```python
from build123d import *

# Parameters (mm, degrees)
EXTRUDE_1_DEPTH      = 3
EXTRUDE_1_DEPTH_BACK = 3
SKETCH_1_W           = 34
SKETCH_1_H           = 70
SKETCH_3_W           = 34
SKETCH_3_H           = 230
EXTRUDE_2_DEPTH      = 5
SKETCH_4_W           = 34
SKETCH_4_H           = 5
EXTRUDE_3_DEPTH      = 30
EXTRUDE_START        = -5
EXTRUDE_4_OUTLINE_W  = 34
EXTRUDE_4_OUTLINE_H  = 25
EXTRUDE_4_DEPTH      = 5
SKETCH_7_R           = 2.2
CUT_EXTRUDE_1_DEPTH  = 139.343774706
SKETCH_9_R           = 3.25
CUT_EXTRUDE_3_DEPTH  = 126.749751491
EXTRUDE_5_DEPTH      = 34
SKETCH_12_W          = 37
SKETCH_12_H          = 52.36766615
CUT_EXTRUDE_5_DEPTH  = 139.343774706
EXTRUDE_START_2      = 3.5
SKETCH_13_W          = 12
SKETCH_13_H          = 10
SKETCH_13_W_2        = 10
SKETCH_13_H_2        = 9
SKETCH_13_R          = 2.2
EXTRUDE_6_DEPTH      = 3.5
EXTRUDE_START_3      = 1.5
SKETCH_14_W          = 10
SKETCH_14_H          = 9
SKETCH_14_R          = 2.2
EXTRUDE_7_DEPTH      = 1.5
SKETCH_15_W          = 7
SKETCH_15_H          = 10
SKETCH_15_R          = 1.9
EXTRUDE_8_DEPTH      = 5
FILLET_2_R           = 15
FILLET_3_R           = 4
FILLET_4_R           = 3
FILLET_5_R           = 6
FILLET_6_R           = 1


# Read off the part's stored shape, not the designer's step: 凸台-拉伸4
with BuildPart() as part:
    # 草图1 → 凸台-拉伸1 (new, two sides: drawn at the far end of the back side and taken through both)
    with BuildSketch(Plane(origin=(0, 0, 0), x_dir=(1, 0, 0), z_dir=(0, 1, 0)).offset(-EXTRUDE_1_DEPTH_BACK)):
        Rectangle(SKETCH_1_W, SKETCH_1_H)
    extrude(amount=EXTRUDE_1_DEPTH + EXTRUDE_1_DEPTH_BACK)

    # 草图3 → 凸台-拉伸2 (add)
    with BuildSketch(Plane.XY.offset(35)):
        Rectangle(SKETCH_3_W, SKETCH_3_H)
    extrude(amount=EXTRUDE_2_DEPTH)

    # 草图4 → 凸台-拉伸3 (add)
    with BuildSketch(Plane.XZ.offset(3)):
        with Locations((0, 7.5)):
            Rectangle(SKETCH_4_W, SKETCH_4_H)
    extrude(amount=EXTRUDE_3_DEPTH)

    # 凸台-拉伸4 outline → 凸台-拉伸4 (add)
    with BuildSketch(Plane.XZ.offset(33).offset(EXTRUDE_START)):
        with Locations((0, 22.5)):
            Rectangle(EXTRUDE_4_OUTLINE_W, EXTRUDE_4_OUTLINE_H)
    extrude(amount=EXTRUDE_4_DEPTH)

    # 草图7 → 切除-拉伸1 (cut, through all)
    with BuildSketch(Plane.XY.offset(40)):
        with Locations((0, -105)):
            Circle(SKETCH_7_R)
        with Locations((0, 105)):
            Circle(SKETCH_7_R)
    extrude(amount=-CUT_EXTRUDE_1_DEPTH, mode=Mode.SUBTRACT)

    # 草图9 → 切除-拉伸3 (cut, through all)
    with BuildSketch(Plane.XZ.offset(3)):
        with Locations(Location((10, -15, 0), (0, 0, 270))):
            Circle(SKETCH_9_R)
        with Locations(Location((-10, -15, 0), (0, 0, 270))):
            Circle(SKETCH_9_R)
    extrude(amount=-CUT_EXTRUDE_3_DEPTH, mode=Mode.SUBTRACT)

    # 草图10 → 凸台-拉伸5 (add)
    with BuildSketch(Plane(origin=(17, 0, 0), x_dir=(0, 0, -1), z_dir=(1, 0, 0))):
        Polygon((-35, 51.819660113), (-35, 63), (-5, 3), (-10.590169944, 3), align=None)
    extrude(amount=-EXTRUDE_5_DEPTH)

    # 草图12 → 切除-拉伸5 (cut, through all)
    with BuildSketch(Plane.XY.offset(40)):
        with Locations((-1.5, -96.183833075)):
            Rectangle(SKETCH_12_W, SKETCH_12_H)
    extrude(amount=-CUT_EXTRUDE_5_DEPTH, mode=Mode.SUBTRACT)

    # 草图13 → 凸台-拉伸6 (add)
    # profile 1 of 3: a face of its own
    with BuildSketch(Plane.XY.offset(40).offset(EXTRUDE_START_2)):
        with Locations((0, -65)):
            Rectangle(SKETCH_13_W, SKETCH_13_H)
    # profile 2 of 3: a face of its own
    with BuildSketch(Plane.XY.offset(40).offset(EXTRUDE_START_2)):
        with Locations((0, 22)):
            Rectangle(SKETCH_13_W, SKETCH_13_H)
    # profile 3 of 3: a face of its own
    with BuildSketch(Plane.XY.offset(40).offset(EXTRUDE_START_2)):
        with Locations((0, 105)):
            Rectangle(SKETCH_13_W_2, SKETCH_13_H_2)
        with Locations((0, 105)):
            Circle(SKETCH_13_R, mode=Mode.SUBTRACT)
    extrude(amount=-EXTRUDE_6_DEPTH)

    # 草图14 → 凸台-拉伸7 (add)
    with BuildSketch(Plane.XY.offset(43.5).offset(EXTRUDE_START_3)):
        with Locations((0, 105)):
            Rectangle(SKETCH_14_W, SKETCH_14_H)
        with Locations((0, 105)):
            Circle(SKETCH_14_R, mode=Mode.SUBTRACT)
    extrude(amount=-EXTRUDE_7_DEPTH)

    # 草图15 → 凸台-拉伸8 (add)
    # profile 1 of 4: a face of its own
    with BuildSketch(Plane.XY.offset(40)):
        with Locations((-9.5, 22)):
            Rectangle(SKETCH_15_W, SKETCH_15_H)
        with Locations((-9.5, 22)):
            Circle(SKETCH_15_R, mode=Mode.SUBTRACT)
    # profile 2 of 4: a face of its own
    with BuildSketch(Plane.XY.offset(40)):
        with Locations((-9.5, -65)):
            Rectangle(SKETCH_15_W, SKETCH_15_H)
        with Locations((-9.5, -65)):
            Circle(SKETCH_15_R, mode=Mode.SUBTRACT)
    # profile 3 of 4: a face of its own
    with BuildSketch(Plane.XY.offset(40)):
        with Locations((9.5, 22)):
            Rectangle(SKETCH_15_W, SKETCH_15_H)
        with Locations(Location((9.5, 22, 0), (0, 0, 180))):
            Circle(SKETCH_15_R, mode=Mode.SUBTRACT)
    # profile 4 of 4: a face of its own
    with BuildSketch(Plane.XY.offset(40)):
        with Locations((9.5, -65)):
            Rectangle(SKETCH_15_W, SKETCH_15_H)
        with Locations(Location((9.5, -65, 0), (0, 0, 180))):
            Circle(SKETCH_15_R, mode=Mode.SUBTRACT)
    extrude(amount=EXTRUDE_8_DEPTH)

    # 圆角2
    fillet_2_edges = [part.edges().sort_by_distance(p)[0] for p in [
        (17, 115, 37.5),
        (-17, 115, 37.5),
        (-17, 0, -35),
        (17, 0, -35),
    ]]
    fillet(fillet_2_edges, radius=FILLET_2_R)

    # 圆角3
    fillet_3_edges = [part.edges().sort_by_distance(p)[0] for p in [
        (-17, -70, 37.5),
        (17, -70, 37.5),
    ]]
    fillet(fillet_3_edges, radius=FILLET_3_R)

    # 圆角4
    fillet_4_edges = [part.edges().sort_by_distance(p)[0] for p in [
        (0, 3, 5),
        (0, 3, 10.590169944),
        (0, 51.819660113, 35),
        (0, 63, 35),
        (0, -3, 35),
        (0, 3, 35),
        (0, -3, 10),
        (0, -28, 10),
        (0, -33, 35),
        (0, -28, 35),
    ]]
    fillet(fillet_4_edges, radius=FILLET_4_R)

    # 圆角5
    fillet_5_edges = [part.edges().sort_by_distance(p)[0] for p in [
        (0, -33, 5),
    ]]
    fillet(fillet_5_edges, radius=FILLET_5_R)

    # 圆角6
    fillet_6_edges = [part.edges().sort_by_distance(p)[0] for p in [
        (5, 100.5, 42.5),
        (5, 109.5, 42.5),
        (-5, 109.5, 42.5),
        (-5, 100.5, 42.5),
        (-13, 27, 42.5),
        (-13, 17, 42.5),
        (-13, -60, 42.5),
        (-13, -70, 42.5),
        (13, 27, 42.5),
        (13, 17, 42.5),
        (13, -70, 42.5),
        (13, -60, 42.5),
    ]]
    fillet(fillet_6_edges, radius=FILLET_6_R)


solid = part.part
```
Here's how the part is built. I have some questions about the finished solid (model axes, mm). A direction names the side the tool comes from. Give positions to 0.01 mm unless a question says otherwise; leave off trailing zeros. Write each loop counter-clockwise with the first axis right and the second up, starting at its lowest first coordinate (ties: lowest second). Pieces come first, ordered by that corner, then holes.
(1) On a 3-axis mill with a long thin cutter (end or side, diameter ignored), from which of +Z, -Z, +X, -X, +Y, -Y can I reach the whole of each face in a straight line? I mean faces 5 (the face through (-0.238, 4.387, 12.915)), 6 (the face through (-13, -65, 42)), 7 (the face through (5, 105, 43)), 8 (the face through (0, -15, 5)). Say none if no direction works.
Output values:
face 5: +X, -X
face 6: +Z, -X, +Y, -Y
face 7: +Z, +X, +Y
face 8: -Z, +X, -X, -Y
(2) Thinking about a two-plate mould opening in X: for faces 1 (the face through (-1.2, 107.1, 45)), 2 (the face through (-10, -65, 40)), 3 (the face through (-6.778, -0.042, -14.577)), 4 (the face through (-12.49, 0.04, -30.72)), which applies, pulls with the +X half, pulls with the -X half, needs draft (parallel to the pull), parting line crosses it, or undercut?
Output values:
face 1: needs draft
face 2: undercut
face 3: undercut
face 4: pulls with the -X half
(3) Imagine slicing it at C-C, the plane x = 0. Count the separate pieces of the cut face and the enclosed holes in it, and give its area (3 significant figures).
Output values:
separate pieces: 2
enclosed holes: 2
area: 2,030 mm2
(4) If I drill on L1, parallel to X at y = -65, z = 41; L2, parallel to Z at x = 5, y = -17.5; L3, parallel to Y at x = 8.5, z = 13.5, over which ranges is the centre line in solid material (lowest first)?
Output values:
L1: x = -13 to -11.4, -7.6 to 7.6, 11.4 to 13
L2: z = 5 to 10, 35 to 40
L3: y = -33 to -28, -3 to 3.72, 8.82 to 20
(5) Imagine slicing it at A-A, the plane z = 37. Write out the boundary of the cut face in (x, y), and give its area (3 significant figures).
Output values:
outline: (-17, -66) arc R4 ccw to (-13, -70) - (13, -70) arc R4 ccw to (17, -66) - (17, 100) arc R15 ccw to (2, 115) - (-2, 115) arc R15 ccw to (-17, 100) - close; hole circle Ø4.4 at (0, 105)
area: 6,170 mm2
(6) Will these pins go through, and if not, where does the flat tip stop? pin 1 (5 mm diameter, centred on x = -6.5, z = 15.5, fed in from -Y); pin 2 (1 mm diameter, centred on x = 12, y = 53, fed in from -Z); pin 3 (6 mm diameter, centred on x = -13, z = 8, fed in from +Y).
Output values:
pin 1: stops at y = -33
pin 2: stops at z = 29.75
pin 3: stops at y = 15
(7) Imagine slicing it at B-B, the plane y = 33. Write out the boundary of the cut face in (x, z), and give its area (3 significant figures).
Output values:
outline: (-17, 20) - (17, 20) - (17, 25.59) - (-17, 25.59) - close; (-17, 35) - (17, 35) - (17, 40) - (-17, 40) - close
area: 360 mm2
(8) Imagine slicing it at D-D, the plane z = 18. Write out the boundary of the cut face in (x, y).
Output values:
outline: (-17, -33) - (17, -33) - (17, -28) - (-17, -28) - close; (-17, -3) - (17, -3) - (17, 3) - (-17, 3) - close; (-17, 17.82) - (17, 17.82) - (17, 29) - (-17, 29) - close
